```python
from build123d import *

# Parameters (mm, degrees)
SKETCH3_W          = 1.27
SKETCH3_H          = 1.4478
SKETCH9_W          = 0.635
SKETCH9_H          = 0.635
CUT_EXTRUDE1_DEPTH = 50.8


with BuildPart() as part:
    # Sweep2: sweep along a path in Sketch2
    with BuildLine(Plane.XY) as sweep2_path:
        Line((0, 0), (53.848, 0))
        ThreePointArc((53.848, 0), (59.236153673, -2.231846327), (61.468, -7.62))
    # Sketch3 → Sweep2 (sweep)
    with BuildSketch(Plane(origin=(0, 0, 0), x_dir=(0, 0, -1), z_dir=(1, 0, 0))):
        Rectangle(SKETCH3_W, SKETCH3_H)
    sweep(path=sweep2_path.line)

    # Sketch9 → Cut-Extrude1 (cut)
    with BuildSketch(Plane.ZY):
        Rectangle(SKETCH9_W, SKETCH9_H)
    extrude(amount=-CUT_EXTRUDE1_DEPTH, mode=Mode.SUBTRACT)


solid = part.part
```
Geometry: final body of the model. Coordinates: model frame, mm. A direction names the side the tool comes from. Round coordinates to 2 decimals unless told otherwise and drop trailing zeros. Order: outer loops, then holes, each group sorted by start corner. A loop starts at its lowest first (then second) coordinate and runs counter-clockwise, first axis right, second up. Notation, with made-up numbers: (58.5, 34) -> (94.5, 34) arc R13 cw to (94.5, 51) -> close; hole circle Ø9 at (-15, -29.5). An arc over 180 degrees is marked (long way). Use CSV: the item, a comma, the result in double quotes. Start each with the question number.
1) First-contact query: pin 1 Ø0.5 at (y, z) = (0, 0) entering from -X; pin 2 Ø2 at (x, y) = (32.5, -1) entering from -Z (3 decimals). Flat tips, straight axial feed; report the tip coordinate or a pass-through.
2) Section A-A (x = 13.5). Return the cut outline in (y, z) (1 decimal).
3) Set-up query: faces 1 (the face through (59.683, -1.655, 0.009)), 2 (the face through (27, -0.724, 0)). Return all of +Z, -Z, +X, -X, +Y, -Y with unobstructed straight access to the full face (end or side cutting, diameter ignored); none if empty.
4) Material intervals for line 1 along Z through (x, y) = (34, 0) (1 decimal); line 2 along Y through (x, z) = (13, -0.2); line 3 along Y through (x, z) = (39.5, -0.45), sorted ascending. Write a range as from..to.
5) Section C-C (y = -4.5). Return the cut outline in (x, z) (3 decimals), and give its area (3 significant figures).
6) Section D-D (y = -1.5). Return the cut outline in (x, z) (3 decimals), and give its area (3 significant figures).
7) Section B-B (z = 0). Return the cut outline in (x, y), and give its area (3 significant figures).
Returned:
1,pin 1,"stops at x = 50.8"
1,pin 2,"stops at z = -0.635"
2,outline,"(-0.7, -0.6) -> (0.7, -0.6) -> (0.7, 0.6) -> (-0.7, 0.6) -> close; hole (-0.3, -0.3) -> (0.3, -0.3) -> (0.3, 0.3) -> (-0.3, 0.3) -> close"
3,face 1,"+Z, -Z, +X, +Y"
3,face 2,"+Z, -Z, -X, -Y"
4,line 1,"z = -0.6..-0.3, 0.3..0.6"
4,line 2,"y = -0.72..-0.32, 0.32..0.72"
4,line 3,"y = -0.72..0.72"
5,outline,"(59.998, -0.635) -> (61.587, -0.635) -> (61.587, 0.635) -> (59.998, 0.635) -> close"
5,area,"2.02 mm²"
6,outline,"(57.026, -0.635) -> (59.52, -0.635) -> (59.52, 0.635) -> (57.026, 0.635) -> close"
6,area,"3.17 mm²"
7,outline,"(0, -0.72) -> (53.85, -0.72) arc R6.9 cw to (60.74, -7.62) -> (62.19, -7.62) arc R8.34 ccw to (53.85, 0.72) -> (0, 0.72) -> (0, 0.32) -> (50.8, 0.32) -> (50.8, -0.32) -> (0, -0.32) -> close"
7,area,"63.0 mm²"
